Design review of the part built by this model. Coordinates are the model's own, in mm. A direction names the side the tool comes from. Coordinates: 2 decimals unless noted, no trailing zeros. Loops run counter-clockwise (first coordinate to the right, second up) from the corner with the lowest first, then second, coordinate; pieces in that order, holes last. Notation, with made-up numbers: M 9,10.5 L 22,10.5 A22 cw 22,24.5 Z; hole C 43.25,87.25 d7. An arc over 180 degrees is marked long. One line per item, written item: value.
Autodesk Inventor part; units mm, degrees
ref_plane "Work Plane1" through (25, 27.275, 0) normal (0, 1, 0) x (-1, 0, 0)
ref_plane "YZ Plane" through (0, 0, 0) normal (1, 0, 0) x (0, 1, 0)
ref_plane "XY Plane" through (0, 0, 0) normal (0, 0, 1) x (1, 0, 0)
sketch "Sketch1" plane through (0, 0, 0) normal (0, 0, 1) x (1, 0, 0)
  circle A0 centre (25, 22.275) radius 1
  circle A1 centre (25, 22.275) radius 5
  circle A2 centre (25, 22.275) radius 1
  point P0 (0, 0)
  dimension "d0" = 10
  dimension "d6" = 2
extrude "Extrusion1" add sketch "Sketch1" along normal blind 30
sketch "Sketch2" plane through (25, 22.275, 30) normal (0, 0, 1) x (1, 0, 0)
  circle A0 centre (0, 0) radius 5
  circle A1 centre (0, 0) radius 2.5
  circle A2 centre (0, 0) radius 1
  point P0 (-25, -22.275)
extrude "Extrusion2" add sketch "Sketch2" along normal blind 16 contours A1
ref_plane "Work Plane1" through (25, 27.275, 0) normal (0, 1, 0) x (-1, 0, 0)
sketch "Sketch4" plane through (25, 27.275, 0) normal (0, 1, 0) x (-1, 0, 0)
  circle A0 centre (0, 5) radius 1
  line L0 (5, 30) -> (-5, 30)
  line L1 (5, 0) -> (-5, 0)
  line L2 (5, 30) -> (-5, 30)
  line L3 (0, 30) -> (5, 30)
  line L4 (0, 30) -> (0, 25)
  point P0 (25, 0)
  dimension "d8" = 2
  dimension "d18" = 5
  dimension "d19" = 5
hole "Hole1" at (25, 27.275, 5) direction (0, -1, 0) diameter 2.2 depth 5 tip angle 118
sketch "Sketch5" plane through (25, 22.275, 46) normal (0, 0, 1) x (1, 0, 0)
  circle A0 centre (0, 0) radius 1
  point P0 (-25, -22.275)
extrude "Extrusion3" add sketch "Sketch5" against normal blind 36
properties part number "acoplador sensor"
(1) We need section A-A on x = 25. State the section outline as (y, z) points (3 decimals), then the cut area to 3 significant figures.
Reply:
outline: M 17.275,0 L 21.275,0 L 21.275,10 L 23.275,10 L 23.275,6.1 L 27.275,6.1 L 27.275,30 L 24.775,30 L 24.775,46 L 19.775,46 L 19.775,30 L 17.275,30 Z; M 23.275,0 L 27.275,0 L 27.275,3.9 L 23.275,3.9 Z
area: 351 mm2
(2) Tool access review of faces 1 (the flat face through (25, 22, 10)), 2 (the cylindrical face through (25.67, 24.74, 4.13)), 3 (the flat face through (26, 25, 30)): name each direction out of +Z, -Z, +X, -X, +Y, -Y from which nothing blocks a thin tool from reaching the whole face with its end or side.
Reply:
face 1: -Z
face 2: +Y
face 3: +Z
(3) Insertion check: pin 1 (1.5 mm diameter, centred on y = 25, z = 38, fed in from -X); pin 2 (6 mm diameter, centred on x = 27.5, z = 34, fed in from +Y) (3 decimals); pin 3 (3 mm diameter, centred on x = 28, z = 8.5, fed in from +Y). Each pin has a flat end and moves straight along its axis. Give the tip position at first contact, or say it passes through.
Reply:
pin 1: stops at x = 23.47
pin 2: stops at y = 24.775
pin 3: stops at y = 27.04
(4) Mouldability with a two-part tool opening along X and no side actions: class faces 4 (the cylindrical face through (23.02, 23.8, 37.89)), 5 (the flat face through (25, 21, 0)), 6 (the cylindrical face through (25.538, 21.432, 4.93)) as released by +X, released by -X, zero draft, split by the parting line, or undercut.
Reply:
face 4: split by the parting line
face 5: zero draft
face 6: undercut
(5) We need section B-B on y = 24. State the section outline as (x, z) points, then the cut area to 3 significant figures.
Reply:
outline: M 20.31,0 L 29.69,0 L 29.69,30 L 26.81,30 L 26.81,46 L 23.19,46 L 23.19,30 L 20.31,30 Z; hole C 25,5 d2.2
area: 336 mm2
(6) To check wall thickness, follow line 1 along Z through (x, y) = (25, 25.15); line 2 along Z through (x, y) = (25, 24.3); line 3 along Z through (x, y) = (28.25, 24.25). State the ranges of each line that lie inside material, in increasing order. Write a range as [from, to].
Reply:
line 1: z = [0, 3.9], [6.1, 30]
line 2: z = [0, 3.9], [6.1, 46]
line 3: z = [0, 30]
(7) We need section D-D on y = 26.5. State the section outline as (x, z) points, then the cut area to 3 significant figures.
Reply:
outline: M 22.33,0 L 27.67,0 L 27.67,30 L 22.33,30 Z; hole C 25,5 d2.2
area: 157 mm2
